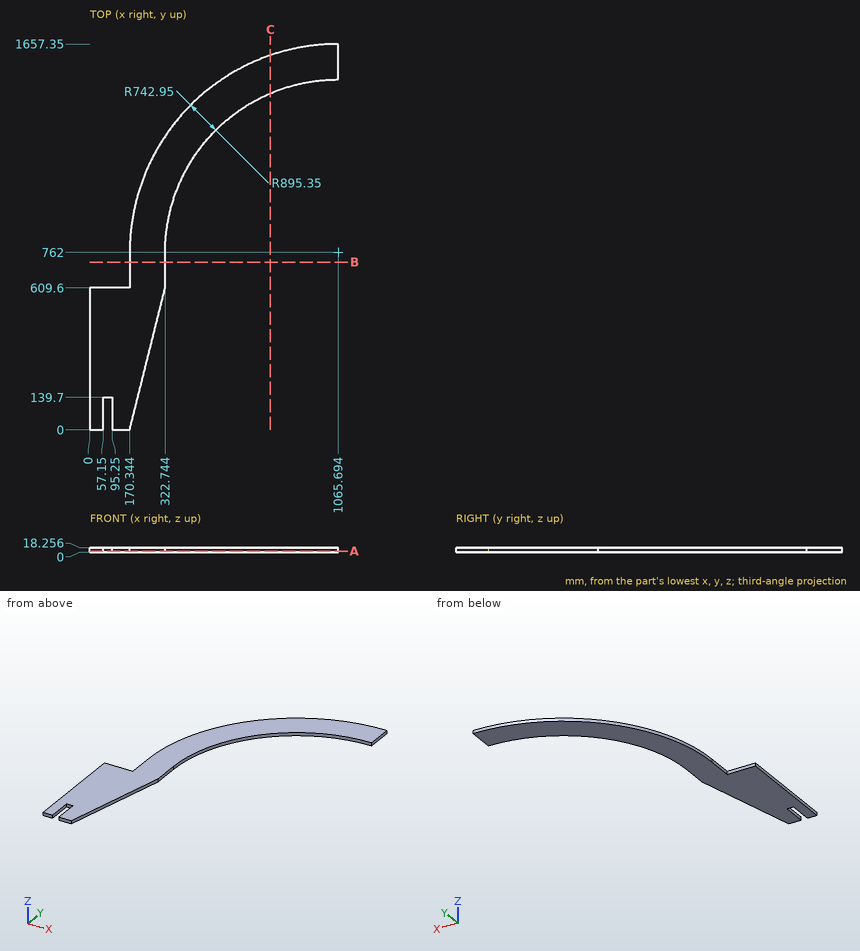
Study the drawing (mm; zero at the part's minimum x, y, z) and answer. Round coordinates to 2 decimals unless told otherwise and drop trailing zeros. Order: outer loops, then holes, each group sorted by start corner. A loop starts at its lowest first (then second) coordinate and runs counter-clockwise, first axis right, second up. Notation, with made-up numbers: M 31.25,64 L 81.25,64 A18 cw 81.25,69 Z; hole C 62.25,61.25 d8. An arc over 180 degrees is marked long. One line per item, written item: value.
Q1. Find section B-B on y = 720. Write down the section's boundary in (x, z), then the cut area to 3 significant figures.
Derived:
outline: M 170.34,0 L 322.74,0 L 322.74,18.26 L 170.34,18.26 Z
area: 2,780 mm²
Q2. Find section C-C on x = 775. Write down the section's boundary in (y, z).
Derived:
outline: M 1445.72,0 L 1608.85,0 L 1608.85,18.26 L 1445.72,18.26 Z
Q3. Find section A-A on z = 4.5. Write down the section's boundary in (x, y), then the cut area to 3 significant figures.
Derived:
outline: M 0,0 L 57.15,0 L 57.15,139.7 L 95.25,139.7 L 95.25,0 L 170.34,0 L 322.74,609.6 L 322.74,762 A742.95 cw 1065.69,1504.95 L 1065.69,1657.35 A895.35 ccw 170.34,762 L 170.34,609.6 L 0,609.6 Z
area: 364,000 mm²
Q4. Flat-ended cylindrical pins translate along their axes: pin 1 (9 mm diameter, centred on x = 126.5, z = 11, fed in from +Y); pin 2 (8 mm diameter, centred on x = 818, z = 15, fed in from +Y); pin 3 (8 mm diameter, centred on y = 460, z = 5.5, fed in from +X). Find the tip coordinate at first contact, or state that the pin passes through.
Derived:
pin 1: y = 609.6
pin 2: y = 1623.55
pin 3: x = 286.34
Q5. Straight lines are drawn through the part: line 1 (Y direction, x = 120, z = 12.25); line 2 (X direction, y = 756, z = 14); line 3 (X direction, y = 88.5, z = 7.25). For each, find the intervals that lie inside material, in ascending order.
Derived:
line 1: 0 to 609.6
line 2: 170.34 to 322.74
line 3: 0 to 57.15, 95.25 to 192.47
